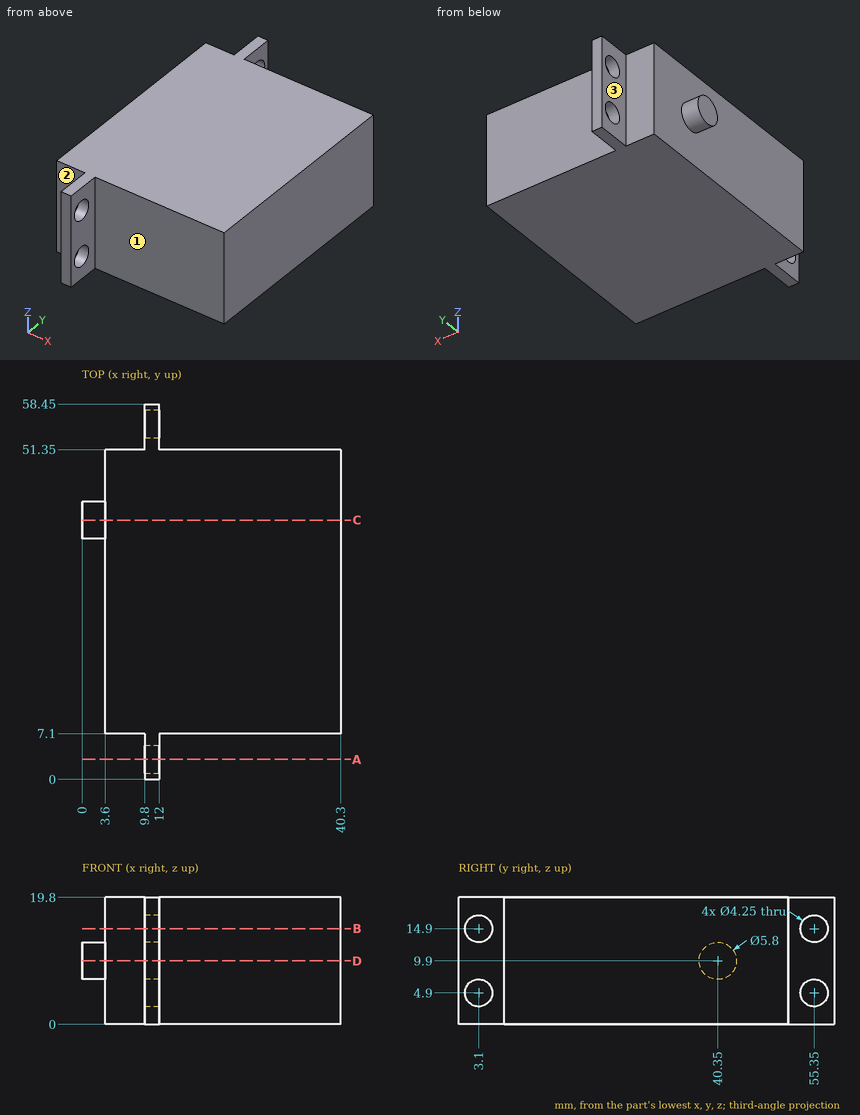
Check sheet for the drawn part. Datum: minimum x, y, z corner. Units: mm. A direction names the side the tool comes from. Round coordinates to 2 decimals unless told otherwise and drop trailing zeros. Loops run counter-clockwise (first coordinate to the right, second up) from the corner with the lowest first, then second, coordinate; pieces in that order, holes last.
Item 1: Access from +Z, -Z, +X, -X, +Y, -Y to the whole of each face (thin tool, end or side, straight path). Record for the marked faces 1, 2 and 3.
Item 2: Gauge pin test, flat ends, axial feed: pin 1 (5 mm diameter, centred on y = 9, z = 2.5, fed in from -X); pin 2 (2 mm diameter, centred on y = 53.5, z = 12, fed in from +X); pin 3 (10 mm diameter, centred on x = 25.5, z = 6, fed in from -Y); pin 4 (6 mm diameter, centred on x = 26.5, y = 12, fed in from -Z). Record the tip position at first contact, or that the pin passes through.
Item 3: Cross-section at D-D on z = 9.9. Record the boundary of the cut face in (x, y).
Item 4: Thickness scan on line 1 (Z direction, x = 10.8, y = 3.1) (3 decimals); line 2 (X direction, y = 49.5, z = 15.5); line 3 (Y direction, x = 4.5, z = 13). Record the ranges inside material, lowest first.
Item 5: Cross-section at A-A on y = 3.1. Record the boundary of the cut face in (x, z) (3 decimals).
Item 6: Cross-section at B-B on z = 14.9. Record the boundary of the cut face in (x, y) (3 decimals), then the cut area to 3 significant figures.
Item 7: Cross-section at C-C on y = 40.35. Record the boundary of the cut face in (x, z).
Answer sheet:
1. face 1: +Z, -Z, +X, -Y
1. face 2: +Z, -Z, -X, -Y
1. face 3: +Z, -Z, -X, +Y
2. pin 1: stops at x = 3.6
2. pin 2: stops at x = 12
2. pin 3: stops at y = 7.1
2. pin 4: stops at z = 0
3. outline: (0, 37.45) - (3.6, 37.45) - (3.6, 7.1) - (9.8, 7.1) - (9.8, 0) - (12, 0) - (12, 7.1) - (40.3, 7.1) - (40.3, 51.35) - (12, 51.35) - (12, 58.45) - (9.8, 58.45) - (9.8, 51.35) - (3.6, 51.35) - (3.6, 43.25) - (0, 43.25) - close
4. line 1: z = 0 to 2.775, 7.025 to 12.775, 17.025 to 19.8
4. line 2: x = 3.6 to 40.3
4. line 3: y = 7.1 to 51.35
5. outline: (9.8, 0) - (12, 0) - (12, 2.775) - (9.8, 2.775) - close; (9.8, 7.025) - (12, 7.025) - (12, 12.775) - (9.8, 12.775) - close; (9.8, 17.025) - (12, 17.025) - (12, 19.8) - (9.8, 19.8) - close
6. outline: (3.6, 7.1) - (9.8, 7.1) - (9.8, 5.225) - (12, 5.225) - (12, 7.1) - (40.3, 7.1) - (40.3, 51.35) - (12, 51.35) - (12, 53.225) - (9.8, 53.225) - (9.8, 51.35) - (3.6, 51.35) - close; (9.8, 0) - (12, 0) - (12, 0.975) - (9.8, 0.975) - close; (9.8, 57.475) - (12, 57.475) - (12, 58.45) - (9.8, 58.45) - close
6. area: 1,640 mm2
7. outline: (0, 7) - (3.6, 7) - (3.6, 0) - (40.3, 0) - (40.3, 19.8) - (3.6, 19.8) - (3.6, 12.8) - (0, 12.8) - close
